```python
from build123d import *

# Parameters (mm, degrees)
BOSS_EXTRUDE1_DEPTH = 3.175
SCREW_HOLES_R       = 1.513296856
SCREW_HOLES_R_2     = 5.08
CUT_EXTRUDE1_DEPTH  = 185.122627276


with BuildPart() as part:
    # Sketch1 → Boss-Extrude1 (new body)
    with BuildSketch(Plane(origin=(0, 0, 0), x_dir=(1, 0, 0), z_dir=(0, 1, 0))):
        with BuildLine():
            Line((-14.549677831, 6.35), (-130.175, 6.35))
            Line((-130.175, 6.35), (-130.175, -6.35))
            Line((-130.175, -6.35), (-14.549677831, -6.35))
            ThreePointArc((-14.549677831, -6.35), (-11.225320151, -11.225320151), (-6.35, -14.549677831))
            Line((-6.35, -14.549677831), (-6.35, -130.175))
            Line((-6.35, -130.175), (6.35, -130.175))
            Line((6.35, -130.175), (6.35, -14.549677831))
            ThreePointArc((6.35, -14.549677831), (11.225320151, -11.225320151), (14.549677831, -6.35))
            Line((14.549677831, -6.35), (130.175, -6.35))
            Line((130.175, -6.35), (130.175, 6.35))
            Line((130.175, 6.35), (14.549677831, 6.35))
            ThreePointArc((14.549677831, 6.35), (0, 15.875), (-14.549677831, 6.35))
        make_face()
    extrude(amount=BOSS_EXTRUDE1_DEPTH)

    # Screw holes → Cut-Extrude1 (cut, through all)
    with BuildSketch(Plane(origin=(0, 0, 0), x_dir=(1, 0, 0), z_dir=(0, 1, 0))):
        with Locations(Location((0, 8, 0), (0, 0, 270))):
            Circle(SCREW_HOLES_R)
        with Locations(Location((0, -8, 0), (0, 0, 270))):
            Circle(SCREW_HOLES_R)
        with Locations(Location((0, 0, 0), (0, 0, 270))):
            Circle(SCREW_HOLES_R_2)
    extrude(amount=CUT_EXTRUDE1_DEPTH, mode=Mode.SUBTRACT)


solid = part.part
```
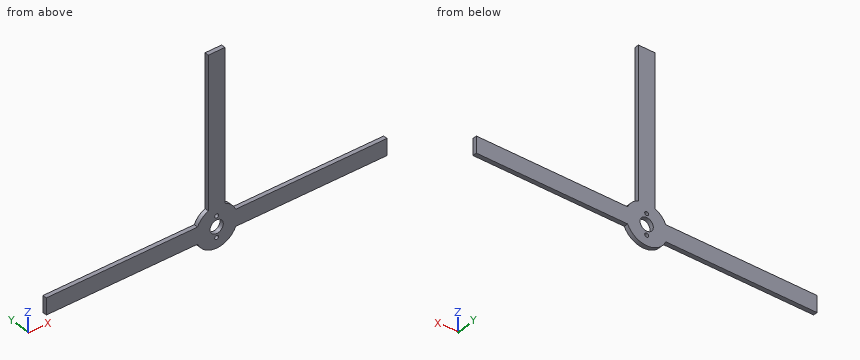
Here's how the part is built. I have some questions about the finished solid (model axes, mm). Round coordinates to 2 decimals unless told otherwise and drop trailing zeros. Order: outer loops, then holes, each group sorted by start corner. A loop starts at its lowest first (then second) coordinate and runs counter-clockwise, first axis right, second up. Notation, with made-up numbers: (11, 6.25) -> (59, 6.25) arc R21 ccw to (59, 24.25) -> close; hole circle Ø4 at (-12, 36). An arc over 180 degrees is marked (long way). Use a Markdown table: item, result. Add a question column.
(1) I need wall thicknesses on line 1 along Z through (x, y) = (0, 1.65) (3 decimals); line 2 along X through (y, z) = (2.5, 0) (3 decimals); line 3 along X through (y, z) = (0.8, 71.5). Which ranges of each line are inside material? Lowest first, please.
(2) Suppose I cut it at B-B, the plane y = 1.65. Please give me the cut outline in (x, z) (3 decimals), and give its area (3 significant figures).
(3) Suppose I cut it at C-C, the plane z = 64. Please give me the cut outline in (x, y) (3 decimals), and give its area (3 significant figures).
(4) Suppose I cut it at D-D, the plane x = -113. Please give me the cut outline in (y, z) (3 decimals).
(5) For pin 1 Ø1.6 at (x, y) = (80.5, 1.5) entering from -Z; pin 2 Ø1 at (y, z) = (1.5, 64.5) entering from -X; pin 3 Ø1 at (x, y) = (-57, 1.5) entering from +Z, each with a flat end and sliding along its axis, tell me the tip position at first contact or that it passes through.
(6) Suppose I cut it at A-A, the plane z = 0. Please give me the cut outline in (x, y) (3 decimals).
Verdict:
| question | item | result |
|---|---|---|
| 1 | line 1 | -15.875 to -9.513, -6.487 to -5.08, 5.08 to 6.487, 9.513 to 130.175 |
| 1 | line 2 | -130.175 to -5.08, 5.08 to 130.175 |
| 1 | line 3 | -6.35 to 6.35 |
| 2 | outline | (-130.175, -6.35) -> (-14.55, -6.35) arc R15.875 ccw to (14.55, -6.35) -> (130.175, -6.35) -> (130.175, 6.35) -> (14.55, 6.35) arc R15.875 ccw to (6.35, 14.55) -> (6.35, 130.175) -> (-6.35, 130.175) -> (-6.35, 14.55) arc R15.875 ccw to (-14.55, 6.35) -> (-130.175, 6.35) -> close; hole circle Ø10.16 at (0, 0); hole circle Ø3.027 at (0, -8); hole circle Ø3.027 at (0, 8) |
| 2 | area | 5,070 mm2 |
| 3 | outline | (-6.35, 0) -> (6.35, 0) -> (6.35, 3.175) -> (-6.35, 3.175) -> close |
| 3 | area | 40.3 mm2 |
| 4 | outline | (0, -6.35) -> (3.175, -6.35) -> (3.175, 6.35) -> (0, 6.35) -> close |
| 5 | pin 1 | z = -6.35 |
| 5 | pin 2 | x = -6.35 |
| 5 | pin 3 | z = 6.35 |
| 6 | outline | (-130.175, 0) -> (-5.08, 0) -> (-5.08, 3.175) -> (-130.175, 3.175) -> close; (5.08, 0) -> (130.175, 0) -> (130.175, 3.175) -> (5.08, 3.175) -> close |
